Autodesk Inventor part; units mm, degrees
ref_plane "YZ Plane" through (0, 0, 0) normal (1, 0, 0) x (0, 1, 0)
ref_plane "XZ Plane" through (0, 0, 0) normal (0, 1, 0) x (-1, 0, 0)
ref_plane "XY Plane" through (0, 0, 0) normal (0, 0, 1) x (1, 0, 0)
sketch "Sketch1" plane through (0, 0, 0) normal (0, 0, 1) x (1, 0, 0)
  circle A0 centre (0, 0) radius 4.5
  circle A1 centre (0, 0) radius 1.5
  dimension "d0" = 9
  dimension "d1" = 3
extrude "Extrusion1" add sketch "Sketch1" along normal mid plane 3
sketch "Sketch2" plane through (0, 0, 1.5) normal (0, 0, 1) x (1, 0, 0)
  circle A0 centre (0, 0) radius 2.1294
  circle A1 centre (0, 0) radius 3.988
extrude "Extrusion2" cut sketch "Sketch2" against normal blind 0.2
mirror "Mirror1" about plane through (0, 0, 0) normal (0, 0, 1) of "Extrusion2"
properties part number "603 Bearing"
CAD build for the part. Positions are in the model's coordinates, mm. A direction names the side the tool comes from. Round coordinates to 2 decimals unless told otherwise and drop trailing zeros. Loops run counter-clockwise (first coordinate to the right, second up) from the corner with the lowest first, then second, coordinate; pieces in that order, holes last. Notation, with made-up numbers: (-12, 40.5) - (22, 40.5) arc R17 cw to (22, 57.5) - close; hole circle Ø6 at (71, 15). An arc over 180 degrees is marked (long way). Put each result on its own line as item: value.
1. Two-plate mould, pull along Y, no slides. Class faces 1 (the flat face through (2, -2, 1.3)), 2 (the cylindrical face through (-0.59, 4.46, 0.02)), 3 (the flat face through (0.9, -1.4, -1.5)), 4 (the cylindrical face through (-1.5, 0.07, 0.02)): released by +Y, released by -Y, zero draft, split by the parting line, or undercut.
Geometry check:
face 1: undercut
face 2: split by the parting line
face 3: zero draft
face 4: undercut
2. Wall check: line 1 (Y direction, x = 0, z = 1.4); line 2 (Y direction, x = 0, z = 0.9); line 3 (Z direction, x = 3, y = 1.25). Give the ranges that are in metal, low to high.
Geometry check:
line 1: -4.5 to -3.99, -2.13 to -1.5, 1.5 to 2.13, 3.99 to 4.5
line 2: -4.5 to -1.5, 1.5 to 4.5
line 3: -1.3 to 1.3
3. Slice it at D-D on y = 3.5. List the corners of the cut face in (x, z), and give its area (3 significant figures).
Geometry check:
outline: (-2.83, -1.5) - (-1.91, -1.5) - (-1.91, -1.3) - (1.91, -1.3) - (1.91, -1.5) - (2.83, -1.5) - (2.83, 1.5) - (1.91, 1.5) - (1.91, 1.3) - (-1.91, 1.3) - (-1.91, 1.5) - (-2.83, 1.5) - close
area: 15.4 mm²
4. Pin check, flat tip, straight feed: P1, Ø1.5, axis at x = 3.5, z = 0, coming from the +Y side. Stop position of the tip, or through.
Geometry check:
P1: y = 3.56
5. Slice it at C-C on z = 0.9. List the corners of the cut face in (x, y), and give its area (3 significant figures).
Geometry check:
outline: circle Ø9 at (0, 0); hole circle Ø3 at (0, 0)
area: 56.5 mm²
6. 3-axis set-ups, long thin cutter, end or side, ignore diameter. For faces 5 (the flat face through (-2, -2, -1.3)), 6 (the flat face through (-3, -3, -1.5)): which of +Z, -Z, +X, -X, +Y, -Y reach the whole face in a straight line?
Geometry check:
face 5: -Z
face 6: -Z, +X, -X, +Y, -Y
7. Slice it at A-A on x = 0. List the corners of the cut face in (y, z).
Geometry check:
outline: (-4.5, -1.5) - (-3.99, -1.5) - (-3.99, -1.3) - (-2.13, -1.3) - (-2.13, -1.5) - (-1.5, -1.5) - (-1.5, 1.5) - (-2.13, 1.5) - (-2.13, 1.3) - (-3.99, 1.3) - (-3.99, 1.5) - (-4.5, 1.5) - close; (1.5, -1.5) - (2.13, -1.5) - (2.13, -1.3) - (3.99, -1.3) - (3.99, -1.5) - (4.5, -1.5) - (4.5, 1.5) - (3.99, 1.5) - (3.99, 1.3) - (2.13, 1.3) - (2.13, 1.5) - (1.5, 1.5) - close
